from build123d import *

# Parameters (mm, degrees)
SKETCH1_W                                           = 150
SKETCH1_H                                           = 105
BOSS_EXTRUDE1_DEPTH                                 = 2
M3_CLEARANCE_HOLE1_AT_2_COUNT                       = 2
M3_CLEARANCE_HOLE1_AT_2_PITCH                       = 120
SKETCH5_R                                           = 14
BOSS_EXTRUDE2_DEPTH                                 = 40
CBORE_FOR_M6_HEX_SOCKET_HEAD_CAP_SCREW1_D           = 6.6
CBORE_FOR_M6_HEX_SOCKET_HEAD_CAP_SCREW1_CBORE_D     = 11
CBORE_FOR_M6_HEX_SOCKET_HEAD_CAP_SCREW1_CBORE_DEPTH = 6.4
FILLET1_R                                           = 1
FILLET2_R                                           = 1
FILLET3_R                                           = 1


with BuildPart() as part:
    # Sketch1 → Boss-Extrude1 (new, symmetric)
    with BuildSketch(Plane.XY):
        Rectangle(SKETCH1_W, SKETCH1_H)
    extrude(amount=BOSS_EXTRUDE1_DEPTH, both=True)

    # Sketch4 → M3 Clearance Hole1 (revolve, cut)
    with BuildSketch(Plane(origin=(60, -37.5, -2), x_dir=(0, 1, 0), z_dir=(1, 0, 0))):
        Polygon((0, 0), (0, 4), (3.3, 4), (1.7, 2.4), (1.7, 0), align=None)
    m3_clearance_hole1 = revolve(axis=Axis((60, -37.5, -8.35), (0, 0, 1)), mode=Mode.SUBTRACT)

    # M3 Clearance Hole1 at 2: M3 Clearance Hole1 ×2
    with Locations(*[(-i * M3_CLEARANCE_HOLE1_AT_2_PITCH, 0, 0) for i in range(1, M3_CLEARANCE_HOLE1_AT_2_COUNT)]):
        add(m3_clearance_hole1, mode=Mode.SUBTRACT)

    # Sketch5 → Boss-Extrude2 (add)
    with BuildSketch(Plane(origin=(0, 0, -2), x_dir=(-1, 0, 0), z_dir=(0, 0, -1))):
        Circle(SKETCH5_R)
    extrude(amount=BOSS_EXTRUDE2_DEPTH)

    # CBORE for M6 Hex Socket Head Cap Screw1 (through all)
    with Locations(Plane.XY.offset(2)):
        with Locations((0, 0)):
            CounterBoreHole(CBORE_FOR_M6_HEX_SOCKET_HEAD_CAP_SCREW1_D / 2, CBORE_FOR_M6_HEX_SOCKET_HEAD_CAP_SCREW1_CBORE_D / 2, CBORE_FOR_M6_HEX_SOCKET_HEAD_CAP_SCREW1_CBORE_DEPTH)

    # Mirror1: M3 Clearance Hole1 across plane
    add(m3_clearance_hole1.mirror(Plane.ZX), mode=Mode.SUBTRACT)

    # Mirror1 copy 1 sketch → Mirror1 copy 1 (revolve, cut)
    with BuildSketch(Plane(origin=(-60, 37.5, -2), x_dir=(0, -1, 0), z_dir=(1, 0, 0))):
        Polygon((0, 0), (0, -4), (3.3, -4), (1.7, -2.4), (1.7, 0), align=None)
    revolve(axis=Axis((-60, 37.5, -8.35), (0, 0, -1)), mode=Mode.SUBTRACT)

    # Fillet1
    fillet1_edges = [part.edges().sort_by_distance(p)[0] for p in [
        (14, 0, -42),
    ]]
    fillet(fillet1_edges, radius=FILLET1_R)

    # Fillet2
    fillet2_edges = [part.edges().sort_by_distance(p)[0] for p in [
        (14, 0, -2),
    ]]
    fillet(fillet2_edges, radius=FILLET2_R)

    # Fillet3
    fillet3_edges = [part.edges().sort_by_distance(p)[0] for p in [
        (75, 0, 2),
        (-75, 0, 2),
    ]]
    fillet(fillet3_edges, radius=FILLET3_R)


solid = part.part
CAD build for the part. Positions are in the model's coordinates, mm. A direction names the side the tool comes from. Coordinates: 2 decimals unless noted, no trailing zeros. Order: outer loops, then holes, each group sorted by start corner. A loop starts at its lowest first (then second) coordinate and runs counter-clockwise, first axis right, second up. Notation, with made-up numbers: (14, 18.5) -> (24, 18.5) arc R31 ccw to (24, 48.5) -> close; hole circle Ø9 at (86, 12). An arc over 180 degrees is marked (long way). Answer in a Markdown table with one row per item.
1) Drill centre lines: line 1 (Y direction, x = 60, z = -1.05); line 2 (X direction, y = 37.5, z = -1.5); line 3 (Y direction, x = 0, z = -15). Where is each one in solid material? Low to high.
Check values:
| item | result |
|---|---|
| line 1 | -52.5 to -39.2, -35.8 to 35.8, 39.2 to 52.5 |
| line 2 | -75 to -61.7, -58.3 to 58.3, 61.7 to 75 |
| line 3 | -14 to -3.3, 3.3 to 14 |
2) Band-saw the part on D-D (y = -43). List the corners of the cut face in (x, z).
Check values:
| item | result |
|---|---|
| outline | (-75, -2) -> (75, -2) -> (75, 1) arc R1 ccw to (74, 2) -> (-74, 2) arc R1 ccw to (-75, 1) -> close |
3) Band-saw the part on C-C (z = -17.5). List the corners of the cut face in (x, y).
Check values:
| item | result |
|---|---|
| outline | circle Ø28 at (0, 0); hole circle Ø6.6 at (0, 0) |
4) Band-saw the part on A-A (x = 60). List the corners of the cut face in (y, z).
Check values:
| item | result |
|---|---|
| outline | (-52.5, -2) -> (-39.2, -2) -> (-39.2, 0.4) -> (-40.8, 2) -> (-52.5, 2) -> close; (-35.8, -2) -> (35.8, -2) -> (35.8, 0.4) -> (34.2, 2) -> (-34.2, 2) -> (-35.8, 0.4) -> close; (39.2, -2) -> (52.5, -2) -> (52.5, 2) -> (40.8, 2) -> (39.2, 0.4) -> close |
5) Mould opens along Y. For faces 1 (the face through (-3, -3, -42)), 2 (the face through (-12.932, -5.362, -21.734)), 3 (the face through (-1, -52.5, 0)), 4 (the face through (4, 0, -4.4)) say: pulls with the +Y half, pulls with the -Y half, needs draft (parallel to the pull), parting line crosses it, or undercut.
Check values:
| item | result |
|---|---|
| face 1 | needs draft |
| face 2 | parting line crosses it |
| face 3 | pulls with the -Y half |
| face 4 | undercut |
6) Which spindle directions (+Z, -Z, +X, -X, +Y, -Y) get a long thin tool onto all of the face, cutting with end or side? Do faces 5 (the face through (-1.19, -5.37, -1.16)), 6 (the face through (2.43, 2.23, -23.46)). Say none if no direction does.
Check values:
| item | result |
|---|---|
| face 5 | +Z |
| face 6 | +Z, -Z |
7) Flat gauge pins, fed straight in: P1, Ø5, axis at y = 23.5, z = -6.5, coming from the -X side; P2, Ø8, axis at y = 13, z = -20, coming from the -X side; P3, Ø1.5, axis at x = 38.5, y = 2, coming from the -Z side; P4, Ø8.5, axis at x = 0, y = 0, coming from the +Z side. Where does each tip first touch, or does it go through?
Check values:
| item | result |
|---|---|
| P1 | through |
| P2 | x = -10.72 |
| P3 | z = -2 |
| P4 | z = -4.4 |
8) Band-saw the part on B-B (y = 37.5). List the corners of the cut face in (x, z), and give its area (3 significant figures).
Check values:
| item | result |
|---|---|
| outline | (-75, -2) -> (-61.7, -2) -> (-61.7, 0.4) -> (-63.3, 2) -> (-74, 2) arc R1 ccw to (-75, 1) -> close; (-58.3, -2) -> (58.3, -2) -> (58.3, 0.4) -> (56.7, 2) -> (-56.7, 2) -> (-58.3, 0.4) -> close; (61.7, -2) -> (75, -2) -> (75, 1) arc R1 ccw to (74, 2) -> (63.3, 2) -> (61.7, 0.4) -> close |
| area | 567 mm2 |
